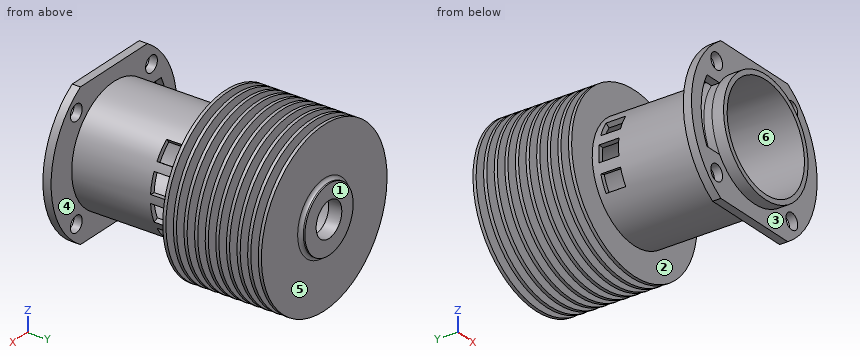
```python
from build123d import *

# Parameters (mm, degrees)
F_3_8_24_TAPPED_HOLE1_D         = 8.4328
CUT_EXTRUDE1_DEPTH              = 6.35
CUT_EXTRUDE2_DEPTH              = 4.7625
F_24_0_152_DIAMETER_HOLE1_D     = 3.8608
F_24_0_152_DIAMETER_HOLE1_DEPTH = 1.984375
CUT_EXTRUDE3_REACH              = 63.361
CUT_EXTRUDE4_REACH              = 63.361


with BuildPart() as part:
    # Sketch1 → Revolve1 (revolve)
    with BuildSketch(Plane.XY, mode=Mode.PRIVATE) as revolve1_sk:
        with BuildLine():
            Line((13.8811, 0), (13.8811, 2.778125))
            Line((13.8811, 2.778125), (20.6375, 2.778125))
            Line((20.6375, 2.778125), (20.6375, 4.7625))
            Line((20.6375, 4.7625), (13.8811, 4.7625))
            Line((13.8811, 4.7625), (13.8811, 31.75))
            Line((13.8811, 31.75), (20.6375, 31.75))
            Line((20.6375, 31.75), (20.6375, 32.512))
            Line((20.6375, 32.512), (13.8811, 32.512))
            Line((13.8811, 32.512), (13.8811, 34.3154))
            Line((13.8811, 34.3154), (20.6375, 34.3154))
            Line((20.6375, 34.3154), (20.6375, 35.0774))
            Line((20.6375, 35.0774), (13.8811, 35.0774))
            Line((13.8811, 35.0774), (13.8811, 36.8808))
            Line((13.8811, 36.8808), (20.6375, 36.8808))
            Line((20.6375, 36.8808), (20.6375, 37.6428))
            Line((20.6375, 37.6428), (13.8811, 37.6428))
            Line((13.8811, 37.6428), (13.8811, 39.4462))
            Line((13.8811, 39.4462), (20.6375, 39.4462))
            Line((20.6375, 39.4462), (20.6375, 40.2082))
            Line((20.6375, 40.2082), (13.8811, 40.2082))
            Line((13.8811, 40.2082), (13.8811, 42.0116))
            Line((13.8811, 42.0116), (20.6375, 42.0116))
            Line((20.6375, 42.0116), (20.6375, 42.7736))
            Line((20.6375, 42.7736), (13.8811, 42.7736))
            Line((13.8811, 42.7736), (13.8811, 44.577))
            Line((13.8811, 44.577), (20.6375, 44.577))
            Line((20.6375, 44.577), (20.6375, 45.339))
            Line((20.6375, 45.339), (13.8811, 45.339))
            Line((13.8811, 45.339), (13.8811, 47.1424))
            Line((13.8811, 47.1424), (20.6375, 47.1424))
            Line((20.6375, 47.1424), (20.6375, 47.9044))
            Line((20.6375, 47.9044), (13.8811, 47.9044))
            Line((13.8811, 47.9044), (13.8811, 49.7078))
            Line((13.8811, 49.7078), (20.6375, 49.7078))
            Line((20.6375, 49.7078), (20.6375, 50.4698))
            Line((20.6375, 50.4698), (13.8811, 50.4698))
            Line((13.8811, 50.4698), (13.8811, 52.2732))
            Line((13.8811, 52.2732), (20.6375, 52.2732))
            Line((20.6375, 52.2732), (20.6375, 53.0352))
            Line((20.6375, 53.0352), (13.8811, 53.0352))
            Line((13.8811, 53.0352), (13.8811, 54.8386))
            Line((13.8811, 54.8386), (20.6375, 54.8386))
            Line((20.6375, 54.8386), (20.6375, 55.6006))
            Line((20.6375, 55.6006), (13.8811, 55.6006))
            Line((13.8811, 55.6006), (8.73125, 55.6006))
            ThreePointArc((8.73125, 55.6006), (8.169983992, 55.833083992), (7.9375, 56.39435))
            Line((7.9375, 56.39435), (7.9375, 56.753125))
            Line((7.9375, 56.753125), (0, 56.753125))
            Line((0, 56.753125), (0, 53.578125))
            Line((0, 53.578125), (12.7, 53.578125))
            Line((12.7, 53.578125), (12.7, 0))
            Line((12.7, 0), (13.8811, 0))
        make_face()
    revolve(revolve1_sk.sketch.rotate(Axis((0, 0, 0), (0, 1, 0)), 90), axis=Axis((0, 0, 0), (0, 1, 0)))

    # 3/8-24 Tapped Hole1 (through all)
    with Locations(Plane(origin=(0, 56.753125, 0), x_dir=(1, 0, 0), z_dir=(0, 1, 0))):
        with Locations((0, 0)):
            Hole(F_3_8_24_TAPPED_HOLE1_D / 2)

    # Sketch4 → Cut-Extrude1 (cut)
    with BuildSketch(Plane(origin=(0, 30.159325, 0), x_dir=(-1, 0, 0), z_dir=(0, -1, 0))):
        with BuildLine():
            Line((-7.840239437, 9.991028254), (-8.569381705, 10.920193881))
            ThreePointArc((-8.569381705, 10.920193881), (-10.315667637, 9.28826886), (-11.756116218, 7.38096665))
            Line((-11.756116218, 7.38096665), (-10.755824536, 6.752942955))
            ThreePointArc((-10.755824536, 6.752942955), (-9.437939284, 8.4979587), (-7.840239437, 9.991028254))
        make_face()
        with BuildLine():
            ThreePointArc((-11.756116218, -7.38096665), (-10.315667637, -9.28826886), (-8.569381705, -10.920193881))
            Line((-8.569381705, -10.920193881), (-7.840239437, -9.991028254))
            ThreePointArc((-7.840239437, -9.991028254), (-9.437939284, -8.4979587), (-10.755824536, -6.752942955))
            Line((-10.755824536, -6.752942955), (-11.756116218, -7.38096665))
        make_face()
        with BuildLine():
            ThreePointArc((-13.845188464, -0.997844484), (-13.468772006, -3.358142025), (-12.693035436, -5.61887788))
            Line((-12.693035436, -5.61887788), (-11.613024187, -5.140784886))
            ThreePointArc((-11.613024187, -5.140784886), (-12.322755724, -3.072408074), (-12.667144066, -0.912940973))
            Line((-12.667144066, -0.912940973), (-13.845188464, -0.997844484))
        make_face()
        with BuildLine():
            ThreePointArc((-12.693035436, 5.61887788), (-13.468772006, 3.358142025), (-13.845188464, 0.997844484))
            Line((-13.845188464, 0.997844484), (-12.667144066, 0.912940973))
            ThreePointArc((-12.667144066, 0.912940973), (-12.322755724, 3.072408074), (-11.613024187, 5.140784886))
            Line((-11.613024187, 5.140784886), (-12.693035436, 5.61887788))
        make_face()
    extrude(amount=CUT_EXTRUDE1_DEPTH, mode=Mode.SUBTRACT)

    # Sketch4<3> → Cut-Extrude2 (cut)
    with BuildSketch(Plane(origin=(0, 30.159325, 0), x_dir=(-1, 0, 0), z_dir=(0, -1, 0))):
        with BuildLine():
            Line((13.218001272, 4.2390305), (12.093322298, 3.878344465))
            ThreePointArc((12.093322298, 3.878344465), (11.414684388, 5.567313564), (10.501569792, 7.141920743))
            Line((10.501569792, 7.141920743), (11.478215783, 7.806119372))
            ThreePointArc((11.478215783, 7.806119372), (12.476250036, 6.085073726), (13.218001272, 4.2390305))
        make_face()
        with BuildLine():
            Line((13.738529509, -1.984375), (12.569560392, -1.81553065))
            ThreePointArc((12.569560392, -1.81553065), (12.7, 0), (12.569560392, 1.81553065))
            Line((12.569560392, 1.81553065), (13.738529509, 1.984375))
            ThreePointArc((13.738529509, 1.984375), (13.8811, 0), (13.738529509, -1.984375))
        make_face()
        with BuildLine():
            Line((11.478215783, -7.806119372), (10.501569792, -7.141920743))
            ThreePointArc((10.501569792, -7.141920743), (11.414684388, -5.567313564), (12.093322298, -3.878344465))
            Line((12.093322298, -3.878344465), (13.218001272, -4.2390305))
            ThreePointArc((13.218001272, -4.2390305), (12.476250036, -6.085073726), (11.478215783, -7.806119372))
        make_face()
    extrude(amount=CUT_EXTRUDE2_DEPTH, mode=Mode.SUBTRACT)

    # #24 (0.152) Diameter Hole1
    with Locations(Plane.XZ.offset(-2.778125)):
        with Locations((-12.347852166, 12.347852166), (12.347852166, 12.347852166), (12.347852166, -12.347852166), (-12.347852166, -12.347852166)):
            Hole(F_24_0_152_DIAMETER_HOLE1_D / 2, depth=F_24_0_152_DIAMETER_HOLE1_DEPTH)

    # Sketch5<2> → Cut-Extrude3 (cut, up to next)
    with BuildSketch(Plane.XZ.offset(-2.778125), mode=Mode.PRIVATE) as cut_extrude3_sk1:
        with BuildLine():
            Line((-10.998522628, 17.4625), (10.998522628, 17.4625))
            ThreePointArc((10.998522628, 17.4625), (0, 20.6375), (-10.998522628, 17.4625))
        make_face()
    cut_extrude3_tool1 = extrude(cut_extrude3_sk1.sketch, amount=-CUT_EXTRUDE3_REACH, mode=Mode.PRIVATE) & part.part
    # Sketch5<2> → Cut-Extrude3 (cut, up to next)
    with BuildSketch(Plane.XZ.offset(-2.778125), mode=Mode.PRIVATE) as cut_extrude3_sk2:
        with BuildLine():
            Line((-10.998522628, -17.4625), (10.998522628, -17.4625))
            ThreePointArc((10.998522628, -17.4625), (0, -20.6375), (-10.998522628, -17.4625))
        make_face()
    cut_extrude3_tool2 = extrude(cut_extrude3_sk2.sketch, amount=-CUT_EXTRUDE3_REACH, mode=Mode.PRIVATE) & part.part
    add(cut_extrude3_tool1.solids().sort_by_distance((0, 2.778125, 18.741265))[0], mode=Mode.SUBTRACT)
    add(cut_extrude3_tool2.solids().sort_by_distance((0, 2.778125, -18.741265))[0], mode=Mode.SUBTRACT)

    # Sketch9 → Cut-Extrude4 (cut, up to next)
    with BuildSketch(Plane.XZ.offset(-2.778125), mode=Mode.PRIVATE) as cut_extrude4_sk1:
        with BuildLine():
            Line((-11.387757943, -7.9375), (-15.554259867, -7.9375))
            ThreePointArc((-15.554259867, -7.9375), (-17.4625, 0), (-15.554259867, 7.9375))
            Line((-15.554259867, 7.9375), (-11.387757943, 7.9375))
            ThreePointArc((-11.387757943, 7.9375), (-13.8811, 0), (-11.387757943, -7.9375))
        make_face()
    cut_extrude4_tool1 = extrude(cut_extrude4_sk1.sketch, amount=-CUT_EXTRUDE4_REACH, mode=Mode.PRIVATE) & part.part
    add(cut_extrude4_tool1.solids().sort_by_distance((-14.932693, 2.778125, 0))[0], mode=Mode.SUBTRACT)


solid = part.part
```
Here's how the part is built. I have some questions about the finished solid (model axes, mm). Face numbers are marked on the shaded views. A direction names the side the tool comes from. Round coordinates to 2 decimals unless told otherwise and drop trailing zeros. Write each loop counter-clockwise with the first axis right and the second up, starting at its lowest first coordinate (ties: lowest second). Pieces come first, ordered by that corner, then holes.
Q1. Which directions (+Z, -Z, +X, -X, +Y, -Y) give clear straight access to the entire face, cutting with the end or side of a thin tool? Please do the marked faces 4, 5 and 6.
Q2. If we section it at B-B on y = 11.5: Write out the boundary of the cut face in (x, z).
Q3. If we mould it in two halves opening along Y, with no side actions, what happens to the marked faces 1, 2 and 3? For each: +Y half, -Y half, draft (parallel to the pull), parting line (faces both ways), or undercut.
Q4. Will these pins go through, and if not, where does the flat tip stop? P1, Ø4, axis at x = 4, z = 9.5, coming from the -Y side; P2, Ø10, axis at x = -7.5, y = 42.5, coming from the +Z side; P3, Ø2, axis at x = -11, z = -6.5, coming from the -Y side; P4, Ø10, axis at y = 25, z = 13.5, coming from the +X side.
Q5. If we section it at A-A on z = 0: Give the number of separate pieces and of enclosed holes in the cut face, plus the area to 3 significant figures.
Q6. Please list where these lines run through material, in increasing order: probe 1 along Y at (x, z) = (-6, -10.5); probe 2 along Z at (x, y) = (1, 46); probe 3 along Z at (x, y) = (-7, 20.5).
Answer below:
1. face 4: none
1. face 5: +Y
1. face 6: -Y
2. outline: circle Ø27.76 at (0, 0); hole circle Ø25.4 at (0, 0)
3. face 1: +Y half
3. face 2: undercut
3. face 3: -Y half
4. P1: stops at y = 53.58
4. P2: stops at z = 20.49
4. P3: stops at y = 0
4. P4: stops at x = 10.86
5. separate pieces: 4
5. enclosed holes: 0
5. area: 292 mm2
6. probe 1: y = 53.58 to 55.6
6. probe 2: z = -13.85 to -12.66, 12.66 to 13.85
6. probe 3: z = -11.99 to -10.6, 10.6 to 11.99
